from build123d import *

# Parameters (mm, degrees)
SKICA1_W                       = 57.8
SKICA1_H                       = 44.4
SKICA1_W_2                     = 55.8
SKICA1_H_2                     = 42.4
VYSUNOUT_TENKOST_NN_1_DEPTH    = 18
SKICA1_2_W                     = 55.8
SKICA1_2_H                     = 42.4
P_IDAT_VYSUNUT_M1_DEPTH        = 1
SKICA2_W                       = 55.8
SKICA2_H                       = 1
ODEBRAT_VYSUNUT_M3_DEPTH       = 13
SKICA3_W                       = 2
SKICA3_H                       = 6
ODEBRAT_VYSUNUT_M4_DEPTH       = 10
SKICA4_W                       = 55.8
SKICA4_H                       = 18
ODEBRAT_VYSUNUT_M5_DEPTH       = 0.4
VYSUNOUT_TENKOST_NN_2_DEPTH    = 18
SKICA5_2_W                     = 20
SKICA5_2_H                     = 23
P_IDAT_VYSUNUT_M2_DEPTH        = 1
SKICA7_W                       = 48
SKICA7_H                       = 23
SKICA7_W_2                     = 46
SKICA7_H_2                     = 21
VYSUNOUT_TENKOST_NN_3_DEPTH    = 18
SKICA7_2_W                     = 46
SKICA7_2_H                     = 21
P_IDAT_VYSUNUT_M3_DEPTH        = 2
SKICA8_W                       = 68
SKICA8_H                       = 24
P_IDAT_VYSUNUT_M4_DEPTH        = 1
SKICA8_2_W                     = 70
SKICA8_2_H                     = 26
SKICA8_2_W_2                   = 68
SKICA8_2_H_2                   = 24
VYSUNOUT_TENKOST_NN_4_DEPTH    = 18
P_IDAT_VYSUNUT_M5_DEPTH        = 18
SKICA10_W                      = 6
SKICA10_H                      = 23
ODEBRAT_VYSUNUT_M7_DEPTH       = 2
SKICA15_W                      = 55.8
SKICA15_H                      = 13
ODEBRAT_VYSUNUT_M13_DEPTH      = 40
SKICA17_W                      = 68
SKICA17_H                      = 20
P_IDAT_VYSUNUT_M6_DEPTH        = 5
P_IDAT_VYSUNUT_M7_DEPTH        = 18
ODEBRAT_VYSUNUT_M14_DEPTH      = 86.4
ODEBRAT_VYSUNUT_M14_DEPTH_BACK = 10
SKICA16_W                      = 12.2
SKICA16_H                      = 13
SKICA19_W                      = 4
SKICA19_H                      = 20
ODEBRAT_VYSUNUT_M15_DEPTH      = 2


with BuildPart() as part:
    # Skica1 → Vysunout tenkost_nn_1 (new body)
    with BuildSketch(Plane.XY):
        with Locations((27.9, 21.2)):
            Rectangle(SKICA1_W, SKICA1_H)
        with Locations((27.9, 21.2)):
            Rectangle(SKICA1_W_2, SKICA1_H_2, mode=Mode.SUBTRACT)
    extrude(amount=VYSUNOUT_TENKOST_NN_1_DEPTH)

    # Skica1_2 → P_idat vysunut_m1 (add)
    with BuildSketch(Plane.XY):
        with Locations((27.9, 21.2)):
            Rectangle(SKICA1_2_W, SKICA1_2_H)
    extrude(amount=P_IDAT_VYSUNUT_M1_DEPTH)

    # Skica2 → Odebrat vysunut_m3 (cut)
    with BuildSketch(Plane.XY.offset(18)):
        with Locations((27.9, -0.5)):
            Rectangle(SKICA2_W, SKICA2_H)
    extrude(amount=-ODEBRAT_VYSUNUT_M3_DEPTH, mode=Mode.SUBTRACT)

    # Skica3 → Odebrat vysunut_m4 (cut)
    with BuildSketch(Plane.ZY.offset(1)):
        with Locations((3.6, 37)):
            Rectangle(SKICA3_W, SKICA3_H)
    extrude(amount=-ODEBRAT_VYSUNUT_M4_DEPTH, mode=Mode.SUBTRACT)

    # Skica4 → Odebrat vysunut_m5 (cut)
    with BuildSketch(Plane.XY.offset(1)):
        with Locations((27.9, 33.4)):
            Rectangle(SKICA4_W, SKICA4_H)
    extrude(amount=-ODEBRAT_VYSUNUT_M5_DEPTH, mode=Mode.SUBTRACT)

    # Skica5 → Vysunout tenkost_nn_2 (add)
    with BuildSketch(Plane.XY):
        Polygon((0, 43.4), (0, 66.4), (20, 66.4), (20, 43.4), (21, 43.4), (21, 67.4), (-1, 67.4), (-1, 43.4), align=None)
    extrude(amount=VYSUNOUT_TENKOST_NN_2_DEPTH)

    # Skica5_2 → P_idat vysunut_m2 (add)
    with BuildSketch(Plane.XY):
        with Locations((10, 54.9)):
            Rectangle(SKICA5_2_W, SKICA5_2_H)
    extrude(amount=P_IDAT_VYSUNUT_M2_DEPTH)

    # Skica7 → Vysunout tenkost_nn_3 (add)
    with BuildSketch(Plane.XY):
        with Locations((44, 54.9)):
            Rectangle(SKICA7_W, SKICA7_H)
        with Locations((44, 54.9)):
            Rectangle(SKICA7_W_2, SKICA7_H_2, mode=Mode.SUBTRACT)
    extrude(amount=VYSUNOUT_TENKOST_NN_3_DEPTH)

    # Skica7_2 → P_idat vysunut_m3 (add)
    with BuildSketch(Plane.XY):
        with Locations((44, 54.9)):
            Rectangle(SKICA7_2_W, SKICA7_2_H)
    extrude(amount=P_IDAT_VYSUNUT_M3_DEPTH)

    # Skica8 → P_idat vysunut_m4 (add)
    with BuildSketch(Plane.XY):
        with Locations((34, 79.4)):
            Rectangle(SKICA8_W, SKICA8_H)
    extrude(amount=P_IDAT_VYSUNUT_M4_DEPTH)

    # Skica8_2 → Vysunout tenkost_nn_4 (add)
    with BuildSketch(Plane.XY):
        with Locations((34, 79.4)):
            Rectangle(SKICA8_2_W, SKICA8_2_H)
        with Locations((34, 79.4)):
            Rectangle(SKICA8_2_W_2, SKICA8_2_H_2, mode=Mode.SUBTRACT)
    extrude(amount=VYSUNOUT_TENKOST_NN_4_DEPTH)

    # Skica9 → P_idat vysunut_m5 (add)
    with BuildSketch(Plane.XY):
        Polygon((71, 92.4), (71, -1), (56.8, -1), (56.8, 43.4), (68, 43.4), (68, 92.4), align=None)
    extrude(amount=P_IDAT_VYSUNUT_M5_DEPTH)

    # Skica10 → Odebrat vysunut_m7 (cut)
    with BuildSketch(Plane(origin=(71, 0, 0), x_dir=(0, 0, -1), z_dir=(1, 0, 0))):
        with Locations((-8, 54.9)):
            Rectangle(SKICA10_W, SKICA10_H)
    extrude(amount=-ODEBRAT_VYSUNUT_M7_DEPTH, mode=Mode.SUBTRACT)

    # Skica15 → Odebrat vysunut_m13 (cut)
    with BuildSketch(Plane.XZ.offset(-42.4)):
        with Locations((27.9, 11.5)):
            Rectangle(SKICA15_W, SKICA15_H)
    extrude(amount=-ODEBRAT_VYSUNUT_M13_DEPTH, mode=Mode.SUBTRACT)

    # Skica17 → P_idat vysunut_m6 (add)
    with BuildSketch(Plane.XY):
        with Locations((34, -11)):
            Rectangle(SKICA17_W, SKICA17_H)
    extrude(amount=P_IDAT_VYSUNUT_M6_DEPTH)

    # Skica18 → P_idat vysunut_m7 (add)
    with BuildSketch(Plane.XY):
        Polygon((-1, -22), (71, -22), (71, -1), (55.8, -1), (55.8, -21), (0, -21), (0, -1), (-1, -1), align=None)
    extrude(amount=P_IDAT_VYSUNUT_M7_DEPTH)

    # Skica16 → Odebrat vysunut_m14 (cut, two sides: drawn at the far end of the back side and taken through both)
    with BuildSketch(Plane.XZ.offset(-65.4).offset(-ODEBRAT_VYSUNUT_M14_DEPTH_BACK)):
        with Locations((61.9, 11.5)):
            Rectangle(SKICA16_W, SKICA16_H)
    extrude(amount=ODEBRAT_VYSUNUT_M14_DEPTH + ODEBRAT_VYSUNUT_M14_DEPTH_BACK, mode=Mode.SUBTRACT)

    # Skica19 → Odebrat vysunut_m15 (cut)
    with BuildSketch(Plane(origin=(69, 0, 0), x_dir=(0, 0, -1), z_dir=(1, 0, 0))):
        with Locations((-8, 55.4)):
            Rectangle(SKICA19_W, SKICA19_H)
    extrude(amount=-ODEBRAT_VYSUNUT_M15_DEPTH, mode=Mode.SUBTRACT)


solid = part.part
Model file for the job. Use its own axes, mm. A direction names the side the tool comes from. Round coordinates to 2 decimals unless told otherwise and drop trailing zeros. Loops run counter-clockwise (first coordinate to the right, second up) from the corner with the lowest first, then second, coordinate; pieces in that order, holes last. Notation, with made-up numbers: (82, -23.5) -> (86, -23.5) arc R15 cw to (86, 4.5) -> close; hole circle Ø11 at (-38, 89.25). An arc over 180 degrees is marked (long way). Answer as CSV lines item,"result". Start each with the question number.
1) Slice it at D-D (y = 58). List the corners of the cut face in (x, z), plus the area to 3 significant figures.
2) Pin check, flat tips, straight feed: P1, Ø5, axis at y = 53.5, z = 6.5, coming from the +X side; P2, Ø23, axis at x = 38, y = 59.5, coming from the +Z side; P3, Ø5.5, axis at x = 24, y = 31, coming from the +Z side; P4, Ø12, axis at x = 41.5, y = 15, coming from the +Z side. Stop position of each tip, or through.
3) Probe line 1 along X through (y, z) = (54, 4); line 2 along Y through (x, z) = (48, 2.25); line 3 along X through (y, z) = (27.5, 7). List the from-to ranges inside material, lowest first.
4) Slice it at C-C (y = -8). List the corners of the cut face in (x, z), plus the area to 3 significant figures.
5) Mould opens along Y. For faces 1 (the face through (71, 34, 9)), 2 (the face through (21, 55, 3)) say: +Y half, -Y half, draft (parallel to the pull), parting line (faces both ways), or undercut.
6) Slice it at B-B (x = 52.5). List the corners of the cut face in (y, z).
7) Tool access for faces 3 (the face through (69, 52.5, 10.7)), 4 (the face through (69, 35, 18)), 5 (the face through (67, 55, 3)): list every direction of +Z, -Z, +X, -X, +Y, -Y with a clear straight run to the whole face (end or side of a thin tool).
8) Slice it at A-A (y = 38.5). List the corners of the cut face in (x, z), plus the area to 3 significant figures.
Filled in:
1,outline,"(-1, 0) -> (71, 0) -> (71, 5) -> (69, 5) -> (69, 6) -> (68, 6) -> (68, 5) -> (67, 5) -> (67, 2) -> (21, 2) -> (21, 5) -> (20, 5) -> (20, 1) -> (0, 1) -> (0, 18) -> (-1, 18) -> close; (68, 10) -> (69, 10) -> (69, 11) -> (71, 11) -> (71, 18) -> (68, 18) -> close"
1,area,"178 mm2"
2,P1,"stops at x = 71"
2,P2,"stops at z = 5"
2,P3,"stops at z = 0.6"
2,P4,"stops at z = 1"
3,line 1,"x = -1 to 0, 20 to 21, 67 to 71"
3,line 2,"y = -22 to 0, 42.4 to 44.4, 65.4 to 67.4, 91.4 to 92.4"
3,line 3,"x = -1 to 0, 68 to 71"
4,outline,"(-1, 0) -> (71, 0) -> (71, 18) -> (68, 18) -> (68, 5) -> (0, 5) -> (0, 18) -> (-1, 18) -> close"
4,area,"412 mm2"
5,face 1,"draft"
5,face 2,"undercut"
6,outline,"(-22, 0) -> (92.4, 0) -> (92.4, 18) -> (91.4, 18) -> (91.4, 1) -> (67.4, 1) -> (67.4, 5) -> (65.4, 5) -> (65.4, 2) -> (44.4, 2) -> (44.4, 5) -> (42.4, 5) -> (42.4, 0.6) -> (24.4, 0.6) -> (24.4, 1) -> (0, 1) -> (0, 5) -> (-21, 5) -> (-21, 18) -> (-22, 18) -> close"
7,face 3,"+X"
7,face 4,"+Z, +X, -X, +Y, -Y"
7,face 5,"+Z"
8,outline,"(-1, 0) -> (71, 0) -> (71, 18) -> (68, 18) -> (68, 5) -> (55.8, 5) -> (55.8, 0.6) -> (0, 0.6) -> (0, 2.6) -> (-1, 2.6) -> close; (-1, 4.6) -> (0, 4.6) -> (0, 18) -> (-1, 18) -> close"
8,area,"164 mm2"
